from build123d import *

# Parameters (mm, degrees)
SKETCH_R           = 18
PAD_DEPTH          = 30
SKETCH001_R        = 14
POCKET_DEPTH       = 20
SKETCH002_R        = 5
PAD001_DEPTH       = 2
SKETCH003_R        = 4
PAD002_DEPTH       = 9
FILLET_R           = 1
SKETCH004_W        = 47.033489
SKETCH004_H        = 47.446069
PAD003_DEPTH       = 10
SKETCH005_W        = 6
SKETCH005_H        = 6
POCKET001_DEPTH    = 15
POLARPATTERN_COUNT = 3
SKETCH006_W        = 48.40057
SKETCH006_H        = 10.44081
POCKET002_DEPTH    = 47.447069
SKETCH007_W        = 8
SKETCH007_H        = 2
POCKET003_DEPTH    = 8


with BuildPart() as part:
    # Sketch → Pad (new body)
    with BuildSketch(Plane.XY):
        Circle(SKETCH_R)
    extrude(amount=PAD_DEPTH)

    # Sketch001 (on Face3 of Pad) → Pocket (cut)
    with BuildSketch(Plane.XY.offset(30)):
        Circle(SKETCH001_R)
    extrude(amount=-POCKET_DEPTH, mode=Mode.SUBTRACT)

    # Sketch002 (on Face5 of Pocket) → Pad001 (join)
    with BuildSketch(Plane.XY.offset(10)):
        Circle(SKETCH002_R)
    extrude(amount=PAD001_DEPTH)

    # Sketch003 (on Face7 of Pad001) → Pad002 (join)
    with BuildSketch(Plane.XY.offset(12)):
        Circle(SKETCH003_R)
    extrude(amount=PAD002_DEPTH)

    # Fillet
    fillet_edges = [part.edges().sort_by_distance(p)[0] for p in [
        (-4, 0, 21),
    ]]
    fillet(fillet_edges, radius=FILLET_R)

    # Sketch004 (on Face8 of Fillet) → Pad003 (join)
    with BuildSketch(Plane.XY.offset(30)):
        with Locations((0.145404, -0.183003)):
            Rectangle(SKETCH004_W, SKETCH004_H)
    extrude(amount=PAD003_DEPTH)

    # Sketch005 (on Face6 of Pad003) → Pocket001 (cut)
    with BuildSketch(Plane.XZ.offset(23.906038)):
        with Locations((-0.069517, 4.047801)):
            Rectangle(SKETCH005_W, SKETCH005_H)
    pocket001 = extrude(amount=-POCKET001_DEPTH, mode=Mode.SUBTRACT)

    # PolarPattern: Pocket001 ×3 about axis
    polarpattern_axis = Axis((0, 0, 0), (0, 0, 1))
    for i in range(1, POLARPATTERN_COUNT):
        add(pocket001.rotate(polarpattern_axis, i * 360 / POLARPATTERN_COUNT), mode=Mode.SUBTRACT)

    # Sketch006 (on Face6 of PolarPattern) → Pocket002 (cut, through all)
    with BuildSketch(Plane.XZ.offset(23.906038)):
        with Locations((0.264744, 35.122468)):
            Rectangle(SKETCH006_W, SKETCH006_H)
    extrude(amount=-POCKET002_DEPTH, mode=Mode.SUBTRACT)

    # Sketch007 (on Face2 of Pocket002) → Pocket003 (cut)
    with BuildSketch(Plane.XY.offset(29.902063)):
        with Locations((0.118946, 15.807168)):
            Rectangle(SKETCH007_W, SKETCH007_H)
    extrude(amount=-POCKET003_DEPTH, mode=Mode.SUBTRACT)


solid = part.part
Geometry check sheet. Reference: the model listing, model coordinates, mm. A direction names the side the tool comes from. Give positions to 0.01 mm unless a question says otherwise; leave off trailing zeros. Loops run counter-clockwise (first coordinate to the right, second up) from the corner with the lowest first, then second, coordinate; pieces in that order, holes last. Notation, with made-up numbers: (20, -19.75) -> (38, -19.75) arc R21 cw to (38, -3.75) -> close; hole circle Ø1 at (53.5, 38). An arc over 180 degrees is marked (long way). Answer in a Markdown table with one row per item. Add a question column.
1) Cross-section at C-C on x = 15.5. Record the boundary of the cut face in (y, z), and give its area (3 significant figures).
2) Material ranges on probe 1 along Y at (x, z) = (0, 17.25); probe 2 along Y at (x, z) = (0, 22.25); probe 3 along Z at (x, y) = (1.5, -13.5), recorded low to high. Write a range as from..to.
3) Cross-section at A-A on z = 11.5. Record the boundary of the cut face in (x, y).
4) Gauge pin test, flat ends, axial feed: P1, Ø1, axis at y = 15.5, z = 27, coming from the -X side; P2, Ø6, axis at x = 14, z = 8, coming from the -Y side; P3, Ø4, axis at x = 13, z = 25.5, coming from the +Y side. Record the tip position at first contact, or that the pin passes through.
5) Draft check along Z on faces 5 (the face through (-0.867, -3.905, 15.944)), 6 (the face through (-10.055, 9.35, 4.006)), 7 (the face through (-12, 7, 1.048)), 8 (the face through (0, 16, 21.902)). Enter one of: pulls with the +Z half, pulls with the -Z half, needs draft (parallel to the pull), parting line crosses it, or undercut.
6) Set-up check for faces 1 (the face through (-12, 7, 7.048)), 2 (the face through (0, 16.807, 26)), 3 (the face through (0, -8.906, 4)), 4 (the face through (10.14, 9.24, 4.01)): record each of +Z, -Z, +X, -X, +Y, -Y from which the full face is reachable in a straight line by a thin tool's end or side.
7) Cross-section at D-D on x = 10.5. Record the boundary of the cut face in (y, z).
8) Cross-section at B-B on y = 0. Record the boundary of the cut face in (x, z).
Outcome:
| question | item | result |
|---|---|---|
| 1 | outline | (-9.15, 0) -> (9.15, 0) -> (9.15, 1.05) -> (5.4, 1.05) -> (5.4, 7.05) -> (9.15, 7.05) -> (9.15, 29.9) -> (-9.15, 29.9) -> close |
| 1 | area | 525 mm^2 |
| 2 | probe 1 | y = -18..-14, -4..4, 14..18 |
| 2 | probe 2 | y = -18..-14, 14..14.81, 16.81..18 |
| 2 | probe 3 | z = 0..1.05, 7.05..10 |
| 3 | outline | circle Ø36 at (0, 0); circle Ø10 at (0, 0); hole circle Ø28 at (0, 0) |
| 4 | P1 | stops at x = -9.95 |
| 4 | P2 | stops at y = -14.25 |
| 4 | P3 | stops at y = 14.25 |
| 5 | face 5 | needs draft |
| 5 | face 6 | undercut |
| 5 | face 7 | undercut |
| 5 | face 8 | pulls with the +Z half |
| 6 | face 1 | none |
| 6 | face 2 | +Z |
| 6 | face 3 | -Y |
| 6 | face 4 | +X |
| 7 | outline | (-14.62, 0) -> (14.62, 0) -> (14.62, 29.9) -> (9.26, 29.9) -> (9.26, 10) -> (-9.26, 10) -> (-9.26, 29.9) -> (-14.62, 29.9) -> close; hole (2.52, 1.05) -> (9.45, 1.05) -> (9.45, 7.05) -> (2.52, 7.05) -> close |
| 8 | outline | (-18, 0) -> (18, 0) -> (18, 29.9) -> (14, 29.9) -> (14, 10) -> (5, 10) -> (5, 12) -> (4, 12) -> (4, 20) arc R1 ccw to (3, 21) -> (-3, 21) arc R1 ccw to (-4, 20) -> (-4, 12) -> (-5, 12) -> (-5, 10) -> (-14, 10) -> (-14, 29.9) -> (-18, 29.9) -> close |
